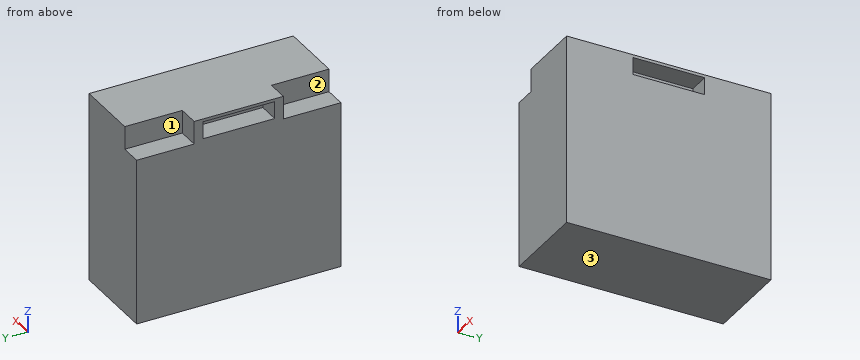
from build123d import *

# Parameters (mm, degrees)
F0_W     = 76.2
F0_H     = 180.34
F1_DEPTH = 167.64
F2_W     = 19.05
F2_H     = 50.8
F3_DEPTH = 20.32
F4_W     = 63.5
F4_H     = 15.24
F5_DEPTH = 19.05
F6_W     = 63.5
F6_H     = 15.24
F7_DEPTH = 19.05


with BuildPart() as f1:
    # F0 (on Top) → F1 (new body)
    with BuildSketch(Plane.XY):
        Rectangle(F0_W, F0_H)
    extrude(amount=F1_DEPTH)

    # F2 (on face) → F3 (cut)
    with BuildSketch(Plane.XY.offset(167.64)):
        with Locations((-28.575, -64.77)):
            Rectangle(F2_W, F2_H)
        with Locations((-28.575, 64.77)):
            Rectangle(F2_W, F2_H)
    extrude(amount=-F3_DEPTH, mode=Mode.SUBTRACT)

    # F4 (on face) → F5 (cut)
    with BuildSketch(Plane(origin=(-38.1, 0, 0), x_dir=(0, -1, 0), z_dir=(-1, 0, 0))):
        with Locations((0, 157.48)):
            Rectangle(F4_W, F4_H)
    extrude(amount=-F5_DEPTH, mode=Mode.SUBTRACT)

    # F6 (on face) → F7 (cut)
    with BuildSketch(Plane.YZ.offset(38.1)):
        with Locations((0, 157.48)):
            Rectangle(F6_W, F6_H)
    extrude(amount=-F7_DEPTH, mode=Mode.SUBTRACT)


solid = f1.part
CAD build for the part. Positions are in the model's coordinates, mm. Face numbers are marked on the shaded views. A direction names the side the tool comes from. Round coordinates to 2 decimals unless told otherwise and drop trailing zeros. Write each loop counter-clockwise with the first axis right and the second up, starting at its lowest first coordinate (ties: lowest second). Pieces come first, ordered by that corner, then holes. Notation, with made-up numbers: M 15.5,35 L 68.5,35 A23 cw 68.5,57 Z; hole C 21.5,-12.75 d1. An arc over 180 degrees is marked long. Use a Markdown table: item, result. Add a question column.
1. Flat gauge pins, fed straight in: P1, Ø5.5, axis at x = -33, y = 66.5, coming from the +Z side; P2, Ø6, axis at y = -68, z = 152.5, coming from the -X side; P3, Ø4.5, axis at x = -28, z = 158, coming from the +Y side. Where does each tip first touch, or does it go through?
2. Drill centre lines: probe 1 along Z at (x, y) = (35, 24); probe 2 along X at (y, z) = (-50, 147.5); probe 3 along Z at (x, y) = (-22.5, 40). Where is each one in solid material? Low to high.
3. Slice it at A-A on z = 155. Give the cut face in (x, y).
4. Slice it at D-D on x = 30. Give the cut face in (y, z).
5. Slice it at C-C on x = -25. Give the cut face in (y, z), then the cut area to 3 significant figures.
6. Slice it at B-B on y = -21. Give the cut face in (x, z).
7. 3-axis set-ups, long thin cutter, end or side, ignore diameter. For the marked faces 1, 2 and 3: which of +Z, -Z, +X, -X, +Y, -Y reach the whole face in a straight line?
Reply:
| question | item | result |
|---|---|---|
| 1 | P1 | stops at z = 147.32 |
| 1 | P2 | stops at x = -19.05 |
| 1 | P3 | stops at y = 39.37 |
| 2 | probe 1 | z = 0 to 149.86, 165.1 to 167.64 |
| 2 | probe 2 | x = -19.05 to 38.1 |
| 2 | probe 3 | z = 0 to 147.32 |
| 3 | outline | M -38.1,-39.37 L -19.05,-39.37 L -19.05,-90.17 L 38.1,-90.17 L 38.1,-31.75 L 19.05,-31.75 L 19.05,31.75 L 38.1,31.75 L 38.1,90.17 L -19.05,90.17 L -19.05,39.37 L -38.1,39.37 L -38.1,31.75 L -19.05,31.75 L -19.05,-31.75 L -38.1,-31.75 Z |
| 4 | outline | M -90.17,0 L 90.17,0 L 90.17,167.64 L -90.17,167.64 Z; hole M -31.75,149.86 L 31.75,149.86 L 31.75,165.1 L -31.75,165.1 Z |
| 5 | outline | M -90.17,0 L 90.17,0 L 90.17,147.32 L 39.37,147.32 L 39.37,167.64 L -39.37,167.64 L -39.37,147.32 L -90.17,147.32 Z; hole M -31.75,149.86 L 31.75,149.86 L 31.75,165.1 L -31.75,165.1 Z |
| 5 | area | 27,200 mm^2 |
| 6 | outline | M -38.1,0 L 38.1,0 L 38.1,149.86 L 19.05,149.86 L 19.05,165.1 L 38.1,165.1 L 38.1,167.64 L -38.1,167.64 L -38.1,165.1 L -19.05,165.1 L -19.05,149.86 L -38.1,149.86 Z |
| 7 | face 1 | +Z, -X, +Y |
| 7 | face 2 | +Z, -X, -Y |
| 7 | face 3 | -Z, +X, -X, +Y, -Y |
